Geometry: final body of the model. Coordinates: model frame, mm. A direction names the side the tool comes from. Round coordinates to 2 decimals unless told otherwise and drop trailing zeros. Order: outer loops, then holes, each group sorted by start corner. A loop starts at its lowest first (then second) coordinate and runs counter-clockwise, first axis right, second up. Notation, with made-up numbers: M -24.75,27.5 L 16.25,27.5 A27 cw 16.25,61.5 Z; hole C 17.25,42.5 d1. An arc over 180 degrees is marked long. Put each result on its own line as item: value. Start each with the question number.
1) Access query for faces 3 (the cylindrical face through (-5.34, 25.83, -5.82)), 4 (the flat face through (-6.965, 11.958, -4.087)), 5 (the flat face through (4, 11.4, 3)). Directions: +Z, -Z, +X, -X, +Y, -Y. A direction counts if a zero-diameter tool reaches every point of the face in a straight line with its end or side. Return the directions, or none.
2) Section B-B, the plane x = 0. Count the separate pieces of the cut face and the enclosed holes in it, then the cut area to 3 significant figures.
3) Material intervals for probe 1 along Y at (x, z) = (1, -5); probe 2 along Y at (x, z) = (5, -7); probe 3 along X at (y, z) = (26.55, 0), sorted ascending. Write a range as [from, to].
4) Section C-C, the plane y = 8.5. Return loops of the section in (x, z) (3 decimals), then the cut area to 3 significant figures.
5) Section A-A, the plane y = 1.65. Return loops of the section in (x, z) (1 decimal), then the cut area to 3 significant figures.
6) Draft query along Y for faces 1 (the flat face through (4, 3.3, -3)), 2 (the flat face through (0, 7, -8.075)). Return one class per face: pulls with the +Y half, pulls with the -Y half, needs draft (parallel to the pull), parting line crosses it, or undercut.
7) First-contact query: P1, Ø2.5, axis at x = 0, z = 0, coming from the -Y side; P2, Ø4, axis at x = 0, y = 19, coming from the +Z side; P3, Ø3, axis at y = 7.5, z = 3, coming from the -X side; P4, Ø4, axis at y = 11, z = 4, coming from the +X side. Flat tips, straight axial feed; report the tip coordinate or a pass-through.
from build123d import *

# Parameters (mm, degrees)
FILLET1_R              = 0.25
SKETCH2_OUTSIDE_W      = 30.044
SKETCH2_OUTSIDE_H      = 30.044
CUT_EXTRUDE1_DEPTH     = 32.905485422
M2_TAPPED_HOLE1_REACH  = 36.101
M2_TAPPED_HOLE1_BORE_R = 0.8
CHAMFER1_SIZE          = 0.25
CHAMFER2_SIZE          = 0.5
CUT_EXTRUDE2_START     = -1
SKETCH6_R              = 7.9
CUT_EXTRUDE2_DEPTH     = 1
SKETCH7_W              = 4
SKETCH7_H              = 1.5


with BuildPart() as part:
    # Sketch1 → Revolve1 (revolve)
    with BuildSketch(Plane(origin=(0, 0, 0), x_dir=(0, 0, -1), z_dir=(1, 0, 0)), mode=Mode.PRIVATE) as revolve1_sk:
        Polygon((3, 0), (3, 3), (1.55, 3), (1.55, 24.1), (2.5, 24.1), (2.5, 28.6), (7.9, 28.6), (7.9, 23.85), (6, 23.85), (6, 19.3), (7.9, 19.3), (7.9, 14.8), (10, 14.8), (10, 13.7), (4.825, 13.7), (4.825, 12.5), (10, 12.5), (10, 11.4), (4.825, 11.4), (4.825, 10.2), (10, 10.2), (10, 9.1), (4.825, 9.1), (4.825, 7.9), (10, 7.9), (10, 6.8), (4.825, 6.8), (4.825, 5.6), (10, 5.6), (10, 4.5), (4.825, 4.5), (4.825, 3.3), (10, 3.3), (10, 0), align=None)
    revolve(revolve1_sk.sketch.rotate(Axis((0, 57.621425894, 0), (0, -1, 0)), 180), axis=Axis((0, 57.621425894, 0), (0, -1, 0)))

    # Fillet1
    fillet1_edges = [part.edges().sort_by_distance(p)[0] for p in [
        (0, 14.8, -7.9),
    ]]
    fillet(fillet1_edges, radius=FILLET1_R)

    # Sketch2 outside → Cut-Extrude1 (cut, through all)
    with BuildSketch(Plane(origin=(0, 28.6, 0), x_dir=(1, 0, 0), z_dir=(0, 1, 0))):
        Rectangle(SKETCH2_OUTSIDE_W, SKETCH2_OUTSIDE_H)
        with BuildLine():
            Line((-4.084753155, -8.075), (4.084753155, -8.075))
            ThreePointArc((4.084753155, -8.075), (4.584753155, -7.941025404), (4.950778558, -7.575))
            Line((4.950778558, -7.575), (9.035531713, -0.5))
            ThreePointArc((9.035531713, -0.5), (9.169506309, 0), (9.035531713, 0.5))
            Line((9.035531713, 0.5), (4.950778558, 7.575))
            ThreePointArc((4.950778558, 7.575), (4.584753155, 7.941025404), (4.084753155, 8.075))
            Line((4.084753155, 8.075), (-4.084753155, 8.075))
            ThreePointArc((-4.084753155, 8.075), (-4.584753155, 7.941025404), (-4.950778558, 7.575))
            Line((-4.950778558, 7.575), (-9.035531713, 0.5))
            ThreePointArc((-9.035531713, 0.5), (-9.169506309, 0), (-9.035531713, -0.5))
            Line((-9.035531713, -0.5), (-4.950778558, -7.575))
            ThreePointArc((-4.950778558, -7.575), (-4.584753155, -7.941025404), (-4.084753155, -8.075))
        make_face(mode=Mode.SUBTRACT)
    extrude(amount=-CUT_EXTRUDE1_DEPTH, mode=Mode.SUBTRACT)

    # M2 Tapped Hole1 bore → M2 Tapped Hole1 (cut, up to next)
    with BuildSketch(Plane.XY.offset(8.075), mode=Mode.PRIVATE) as m2_tapped_hole1_sk1:
        with Locations((0, 1.65)):
            Circle(M2_TAPPED_HOLE1_BORE_R)
    m2_tapped_hole1_tool1 = extrude(m2_tapped_hole1_sk1.sketch, amount=-M2_TAPPED_HOLE1_REACH, mode=Mode.PRIVATE) & part.part
    add(m2_tapped_hole1_tool1.solids().sort_by_distance((0, 1.65, 8.075))[0], mode=Mode.SUBTRACT)

    # Chamfer1
    chamfer1_edges = [part.edges().sort_by_distance(p)[0] for p in [
        (0, 19.3, -7.9),
        (0, 23.85, -7.9),
        (0, 28.6, -7.9),
    ]]
    chamfer(chamfer1_edges, length=CHAMFER1_SIZE)

    # Chamfer2
    chamfer2_edges = [part.edges().sort_by_distance(p)[0] for p in [
        (0, 28.6, -2.5),
    ]]
    chamfer(chamfer2_edges, length=CHAMFER2_SIZE)

    # Sketch6 → Cut-Extrude2 (cut)
    with BuildSketch(Plane(origin=(0, 28.6, 0), x_dir=(1, 0, 0), z_dir=(0, 1, 0)).offset(CUT_EXTRUDE2_START)):
        with Locations(Location((0, 0, 0), (0, 0, 270))):
            Circle(SKETCH6_R)
    extrude(amount=CUT_EXTRUDE2_DEPTH, mode=Mode.SUBTRACT)

    # Sketch7 → Cut-Revolve1 (revolve, cut)
    with BuildSketch(Plane(origin=(0, 0, 0), x_dir=(0, 0, -1), z_dir=(1, 0, 0))):
        with Locations((8, 18.55)):
            Rectangle(SKETCH7_W, SKETCH7_H)
    revolve(axis=Axis((0, 0, 0), (0, 1, 0)), mode=Mode.SUBTRACT)


solid = part.part
Result sheet:
1. face 3: +Y
1. face 4: -Z, -X, +Y, -Y
1. face 5: none
2. separate pieces: 3
2. enclosed holes: 0
2. area: 270 mm2
3. probe 1: y = [0, 3.3], [4.5, 5.6], [6.8, 7.9], [9.1, 10.2], [11.4, 12.5], [13.7, 27.6]
3. probe 2: y = [0, 3.3], [4.5, 5.6], [6.8, 7.9], [9.1, 10.2], [11.4, 12.5], [13.7, 14.8]
3. probe 3: x = [-7.9, -2.5], [2.5, 7.9]
4. outline: C 0,0 d9.65; hole C 0,0 d3.1
4. area: 65.6 mm2
5. outline: M -9,-0.5 L -5,-7.6 A1 ccw -4.1,-8.1 L 4.1,-8.1 A1 ccw 5,-7.6 L 9,-0.5 A1 ccw 9,0.5 L 5,7.6 A1 ccw 4.1,8.1 L 0.8,8.1 L 0.8,2.9 A3 cw long -0.8,2.9 L -0.8,8.1 L -4.1,8.1 A1 ccw -5,7.6 L -9,0.5 A1 ccw Z
5. area: 189 mm2
6. face 1: undercut
6. face 2: needs draft
7. P1: passes through
7. P2: stops at z = 7.9
7. P3: stops at x = -8.46
7. P4: stops at x = 8.15
